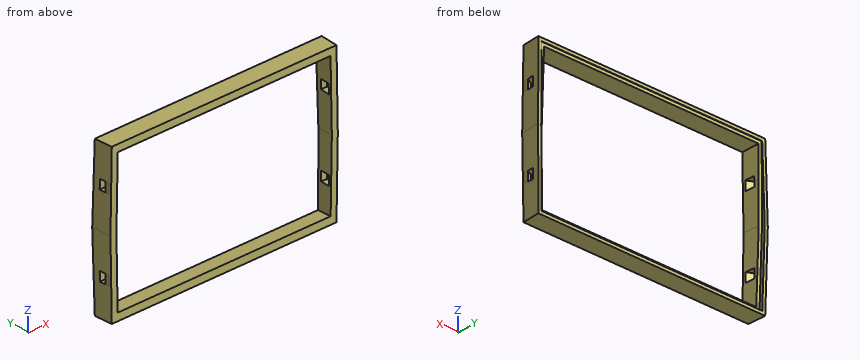
```python
from build123d import *

# Parameters (mm, degrees)
EXTRUDE_1_DEPTH          = 24.5
EXTRUDE_1_DRAFT          = -1
CUT_EXTRUDE_1_REACH      = 120.659
CUT_EXTRUDE_1_DRAFT      = -3
CUT_EXTRUDE_5_DEPTH      = 1
CUT_EXTRUDE_6_DEPTH      = 3
EXTRUDE_2_DEPTH          = 3
MIRROR_6_COPY_1_DEPTH    = 3
MIRROR_6_COPY_2_DEPTH    = 3
SKETCH_16_W              = 97.890152637
SKETCH_16_H              = 76.040955573
CUT_EXTRUDE_7_DEPTH      = 20
CUT_EXTRUDE_7_DEPTH_BACK = 109.33314876


with BuildPart() as part:
    # Sketch 1 → Extrude 1 (with draft: the straight prism first)
    with BuildSketch(Plane.XY):
        Polygon((16.715993843, 25.667879294), (20.215993843, -31.556614873), (87.215993843, -31.556614873), (90.715993843, 25.667879294), align=None)
    extrude(amount=EXTRUDE_1_DEPTH)
    # Extrude 1: the draft: its side faces are tilted about the plane it starts from
    extrude_1_sides = [part.faces().sort_by_distance(p)[0] for p in [
        (18.465993843, -2.94436779, 12.25),
        (53.715993843, -31.556614873, 12.25),
        (88.965993843, -2.94436779, 12.25),
        (53.715993843, 25.667879294, 12.25),
    ]]
    draft(extrude_1_sides, Plane.XY, EXTRUDE_1_DRAFT)

    # Mirror 3: part across plane


with BuildPart() as part_1:
    add(part.part)
    add(part.part.mirror(Plane.XY.offset(24.5)))

    # Cut-Extrude 1: up to this plane
    cut_extrude_1_end = Plane(origin=(20.215993843, -29.556919482, 0.034904813), z_dir=(0, -0.9998476951563913, -0.01745240643728355))



with BuildPart() as cut_extrude_1_long_prism_1:
    # Sketch 2 → Cut-Extrude 1 (the long prism of profile 1, to be tilted and cut off)
    with BuildSketch(Plane(origin=(0, 25.660061204, -0.447898034), x_dir=(1, 0, 0), z_dir=(0, 0.9998476951563913, -0.01745240643728355))):
        Polygon((18.678866318, -47.440503324), (88.753121369, -47.440503324), (89.170598215, -24.951698299), (88.753098752, -2.447966262), (18.678888935, -2.447966262), (18.261389472, -24.951698299), align=None)
    extrude(amount=-CUT_EXTRUDE_1_REACH)
    cut_extrude_1_tool1_sides = [cut_extrude_1_long_prism_1.faces().sort_by_distance(p)[0] for p in [
        (53.715993843, -33.832299375, 48.038274826),
        (88.961859792, -34.028541258, 36.79558489),
        (88.961848484, -34.42115528, 14.302742649),
        (53.715993843, -34.617527418, 3.052590344),
        (18.470139203, -34.42115528, 14.302742649),
        (18.470127895, -34.028541258, 36.79558489),
    ]]
    draft(cut_extrude_1_tool1_sides, Plane(origin=(0, 25.660061204, -0.447898034), x_dir=(1, 0, 0), z_dir=(0, 0.9998476951563913, -0.01745240643728355)), CUT_EXTRUDE_1_DRAFT)  # the draft: side faces tilted about the start plane


with BuildPart() as part_2:
    add(part_1.part)
    cut_extrude_1_tool1 = split(cut_extrude_1_long_prism_1.part, bisect_by=cut_extrude_1_end, keep=Keep.BOTH, mode=Mode.PRIVATE)
    add(cut_extrude_1_tool1.solids().sort_by_distance((53.715994, 26.095398, 24.492555))[0], mode=Mode.SUBTRACT)

    # Sketch 10 → Cut-Extrude 5 (cut)
    with BuildSketch(Plane(origin=(0, 25.660061204, -0.447898034), x_dir=(1, 0, 0), z_dir=(0, 0.9998476951563913, -0.01745240643728355))):
        Polygon((17.697441389, -1.447966262), (89.734546298, -1.447966262), (90.170598215, -24.951698299), (89.714394373, -48.419962311), (17.717593314, -48.419962311), (17.261389472, -24.951698299), align=None)
    extrude(amount=-CUT_EXTRUDE_5_DEPTH, mode=Mode.SUBTRACT)

    # Sketch 13 → Cut-Extrude 6 (cut, symmetric)
    with BuildSketch(Plane(origin=(87.093192584, -4.592650432, -1.535873606), x_dir=(0.017583201594826382, -0.0009272079251698135, 0.999844973636983), z_dir=(-0.998457718176913, 0.05265127083073426, 0.017607631665297937))):
        Polygon((14.826718303, 28.545615626), (14.87901891, 25.545615626), (11.87901891, 25.493315019), (11.826718303, 28.493315019), align=None)
    cut_extrude_6 = extrude(amount=CUT_EXTRUDE_6_DEPTH, both=True, mode=Mode.SUBTRACT)

    # Sketch 14 → Extrude 2 (add)
    with BuildSketch(Plane(origin=(0.283433717, 0.252501642, 15.317338252), x_dir=(-0.9998288893890833, 0.00030489955637755267, 0.018495917907816833), z_dir=(-0.018498430825131588, -0.016479634824702716, -0.9996930677428209))):
        Polygon((-88.431728934, 20.680996021), (-90.383068209, 20.578695502), (-90.452019303, 21.71033965), align=None)
    extrude_2 = extrude(amount=EXTRUDE_2_DEPTH)

    # Mirror 4: Cut-Extrude 6, Extrude 2 across plane
    add(cut_extrude_6.mirror(Plane(origin=(53.715993843, 0, 0), x_dir=(0, 0, 1), z_dir=(1, 0, 0))), mode=Mode.SUBTRACT)
    add(extrude_2.mirror(Plane(origin=(53.715993843, 0, 0), x_dir=(0, 0, 1), z_dir=(1, 0, 0))))

    # Mirror 6: Cut-Extrude 6, Extrude 2 across plane
    add(cut_extrude_6.mirror(Plane.XY.offset(24.5)), mode=Mode.SUBTRACT)
    add(extrude_2.mirror(Plane.XY.offset(24.5)))

    # Mirror 6 copy 1 sketch → Mirror 6 copy 1 (cut, symmetric)
    with BuildSketch(Plane(origin=(20.338795103, -4.592650432, 50.535873606), x_dir=(-0.017583201594826382, -0.0009272079251698135, -0.999844973636983), z_dir=(0.998457718176913, 0.05265127083073426, -0.017607631665297937))):
        Polygon((14.826718303, 28.545615626), (14.87901891, 25.545615626), (11.87901891, 25.493315019), (11.826718303, 28.493315019), align=None)
    extrude(amount=MIRROR_6_COPY_1_DEPTH, both=True, mode=Mode.SUBTRACT)

    # Mirror 6 copy 2 sketch → Mirror 6 copy 2 (add)
    with BuildSketch(Plane(origin=(107.14855397, 0.252501642, 33.682661748), x_dir=(0.9998288893890833, 0.00030489955637755267, -0.018495917907816833), z_dir=(0.018498430825131588, -0.016479634824702716, 0.9996930677428209))):
        Polygon((-88.431728934, 20.680996021), (-90.383068209, 20.578695502), (-90.452019303, 21.71033965), align=None)
    extrude(amount=MIRROR_6_COPY_2_DEPTH)

    # Sketch 16 → Cut-Extrude 7 (cut, two sides)
    with BuildSketch(Plane(origin=(0, 0, 0), x_dir=(1, 0, 0), z_dir=(0, 1, 0))) as cut_extrude_7_sk:
        with Locations((56.945180684, -27.590511427)):
            Rectangle(SKETCH_16_W, SKETCH_16_H)
    extrude(amount=CUT_EXTRUDE_7_DEPTH, mode=Mode.SUBTRACT)
    extrude(cut_extrude_7_sk.sketch, amount=-CUT_EXTRUDE_7_DEPTH_BACK, mode=Mode.SUBTRACT)


solid = part_2.part
```
Input: part model. Units: mm. Frame: model coordinates. Give positions to 0.01 mm unless a question says otherwise; leave off trailing zeros. Order: outer loops, then holes, each group sorted by start corner. A loop starts at its lowest first (then second) coordinate and runs counter-clockwise, first axis right, second up. Notation, with made-up numbers: M 65.25,86.5 L 116.25,86.5 A14 ccw 116.25,110.5 Z; hole C 72.25,6.25 d1. An arc over 180 degrees is marked long. One line per question, with ' | ' between items.
1) Section B-B on z = 32.5. Output: boundary loops of the cut face in (x, y).
Filled in:
outline: M 16.41,25.96 L 16.77,20 L 18.73,20 L 18.46,25.24 L 17.42,25.24 L 17.42,25.96 Z; M 88.7,20 L 90.66,20 L 91.02,25.96 L 90.02,25.96 L 90.02,25.24 L 88.97,25.24 Z
2) Ray query, L1, parallel to X at y = 20.5, z = 19; L2, parallel to X at y = 24.25, z = 8; L3, parallel to Z at x = 68, y = 24.25. Return the intervals inside material, ascending.
Filled in:
L1: x = 16.7 to 18.65, 88.78 to 90.73 | L2: x = 16.66 to 18.65, 88.78 to 90.77 | L3: z = 0 to 2.1, 46.91 to 49
3) Contact query for a flat-ended pin moving along its axis: P1, Ø1.5, axis at y = 24, z = 22, coming from the -X side. Output: stop coordinate, or through.
Filled in:
P1: stops at x = 16.39
4) Section A-A on x = 61. Output: boundary loops of the cut face in (y, z), and give its area (3 significant figures).
Filled in:
outline: M 20,0 L 25.67,0 L 25.69,1 L 24.69,1.02 L 24.7,2.07 L 20,2.4 Z; M 20,46.76 L 25.49,46.95 L 25.51,47.98 L 25.69,47.98 L 25.67,49 L 20,49 Z | area: 23.5 mm2
